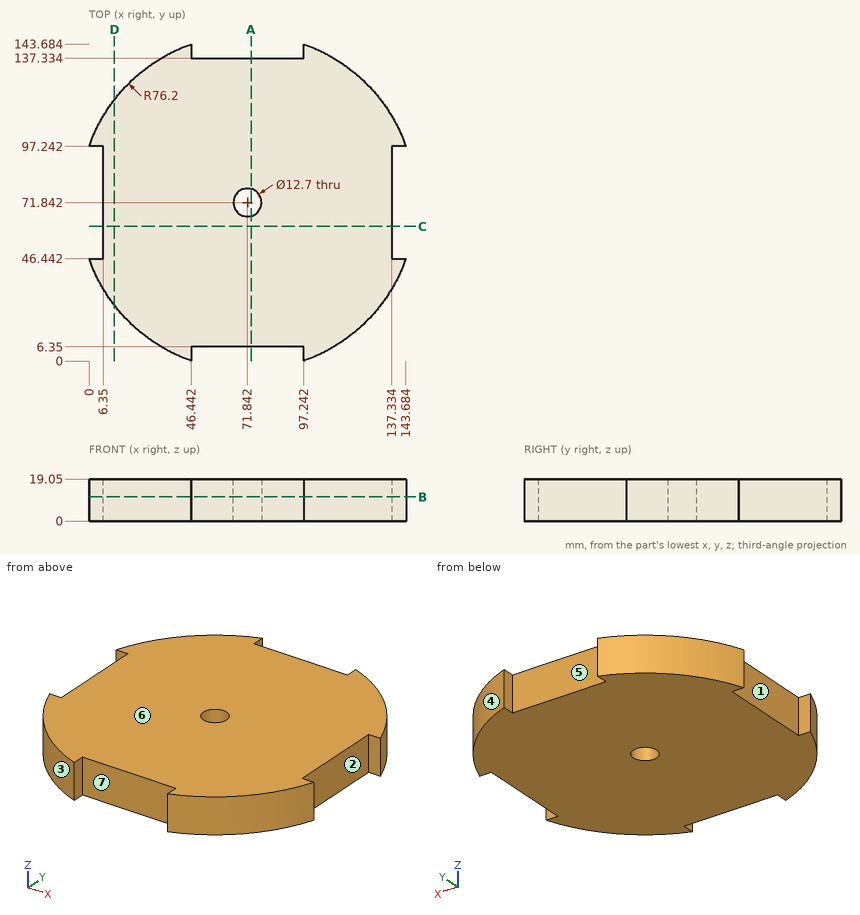
Job drawing, mm, ordinate dimensions from the low corner. One solid piece. A direction names the side the tool comes from. Give positions to 0.01 mm unless a question says otherwise; leave off trailing zeros. Write each loop counter-clockwise with the first axis right and the second up, starting at its lowest first coordinate (ties: lowest second). Pieces come first, ordered by that corner, then holes. Notation, with made-up numbers: (-4, 39) - (41, 39) arc R8 cw to (41, 53) - close; hole circle Ø9 at (31, 6). An arc over 180 degrees is marked (long way). Use one line per item in the form item = value. Start each with the question number.
1. Two-plate mould, pull along X, no slides. Class the marked faces 4, 5, 6 and 7: released by +X, released by -X, zero draft, split by the parting line, or undercut.
2. Band-saw the part on D-D on x = 11.5. Write the cut outline in (y, z), plus the area to 3 significant figures.
3. 3-axis set-ups, long thin cutter, end or side, ignore diameter. For the marked faces 1, 2 and 3: which of +Z, -Z, +X, -X, +Y, -Y reach the whole face in a straight line?
4. Band-saw the part on A-A on x = 73.5. Write the cut outline in (y, z), plus the area to 3 significant figures.
5. Drop flat-ended pins along their axis: pin 1 Ø7 at (x, z) = (2, 8.5) entering from -Y; pin 2 Ø9.5 at (x, z) = (65, 10.5) entering from -Y; pin 3 Ø9.5 at (y, z) = (64, 7) entering from +X; pin 4 Ø8 at (x, z) = (94, 17) entering from -Y. Give the stop position or say it passes through.
6. Probe line 1 (Y direction, x = 48, z = 3.25); line 2 (X direction, y = 73, z = 14). List the from-to ranges inside material, lowest first. Write a range as [from, to].
7. Band-saw the part on B-B on z = 11. Write the cut outline in (x, y), plus the area to 3 significant figures.
8. Band-saw the part on C-C on y = 61. Write the cut outline in (x, z), plus the area to 3 significant figures.
Conclusion:
q1.face_4 = released by +X
q1.face_5 = undercut
q1.face_6 = zero draft
q1.face_7 = undercut
q2.outline = (25.31, 0) - (118.37, 0) - (118.37, 19.05) - (25.31, 19.05) - close
q2.area = 1,770 mm²
q3.face_1 = +Z, -Z, -X
q3.face_2 = +Z, -Z, +X
q3.face_3 = +Z, -Z, -X, -Y
q4.outline = (6.35, 0) - (65.71, 0) - (65.71, 19.05) - (6.35, 19.05) - close; (77.97, 0) - (137.33, 0) - (137.33, 19.05) - (77.97, 19.05) - close
q4.area = 2,260 mm²
q5.pin_1 = 34.36
q5.pin_2 = 6.35
q5.pin_3 = 137.33
q5.pin_4 = 0
q6.line_1 = [6.35, 137.33]
q6.line_2 = [6.35, 65.6], [78.09, 137.33]
q7.outline = (0, 46.44) arc R76.2 ccw to (46.44, 0) - (46.44, 6.35) - (97.24, 6.35) - (97.24, 0) arc R76.2 ccw to (143.68, 46.44) - (137.33, 46.44) - (137.33, 97.24) - (143.68, 97.24) arc R76.2 ccw to (97.24, 143.68) - (97.24, 137.33) - (46.44, 137.33) - (46.44, 143.68) arc R76.2 ccw to (0, 97.24) - (6.35, 97.24) - (6.35, 46.44) - close; hole circle Ø12.7 at (71.84, 71.84)
q7.area = 16,200 mm²
q8.outline = (6.35, 0) - (137.33, 0) - (137.33, 19.05) - (6.35, 19.05) - close
q8.area = 2,500 mm²
